```python
from build123d import *

# Parameters (mm, degrees)
SKETCH3_W           = 50
SKETCH3_H           = 100
BOSS_EXTRUDE1_DEPTH = 8
SKETCH3_3_R         = 8
SKETCH3_3_R_2       = 1.5
CUT_EXTRUDE2_DEPTH  = 10
SKETCH4_R           = 18.5
CUT_EXTRUDE3_DEPTH  = 4


with BuildPart() as part:
    # Sketch3 → Boss-Extrude1 (new body)
    with BuildSketch(Plane.XY):
        with Locations((0, 50)):
            Rectangle(SKETCH3_W, SKETCH3_H)
    extrude(amount=BOSS_EXTRUDE1_DEPTH)

    # Sketch3_3 → Cut-Extrude2 (cut)
    with BuildSketch(Plane.XY):
        with Locations(Location((0, 12.8, 0), (0, 0, 180))):
            Circle(SKETCH3_3_R)
        with Locations(Location((-7.75, 33.223393759, 0), (0, 0, 180))):
            Circle(SKETCH3_3_R_2)
        with Locations(Location((7.75, 33.223393759, 0), (0, 0, 180))):
            Circle(SKETCH3_3_R_2)
        with Locations(Location((-15.5, 19.8, 0), (0, 0, 180))):
            Circle(SKETCH3_3_R_2)
        with Locations(Location((-7.75, 6.376606241, 0), (0, 0, 180))):
            Circle(SKETCH3_3_R_2)
        with Locations(Location((7.75, 6.376606241, 0), (0, 0, 180))):
            Circle(SKETCH3_3_R_2)
        with Locations(Location((15.5, 19.8, 0), (0, 0, 180))):
            Circle(SKETCH3_3_R_2)
    extrude(amount=CUT_EXTRUDE2_DEPTH, mode=Mode.SUBTRACT)

    # Sketch4 → Cut-Extrude3 (cut)
    with BuildSketch(Plane.XY.offset(8)):
        with Locations((0, 19.8)):
            Circle(SKETCH4_R)
    extrude(amount=-CUT_EXTRUDE3_DEPTH, mode=Mode.SUBTRACT)


solid = part.part
```
CAD build for the part. Positions are in the model's coordinates, mm. A direction names the side the tool comes from. Round coordinates to 2 decimals unless told otherwise and drop trailing zeros. Loops run counter-clockwise (first coordinate to the right, second up) from the corner with the lowest first, then second, coordinate; pieces in that order, holes last. Notation, with made-up numbers: M -27,-33 L -11,-33 A12 cw -11,-29 Z; hole C -23,-10 d1. An arc over 180 degrees is marked long. Return JSON: item names as keys, results as strings. Group by question number.
(1) Saw through at A-A, the plane x = -15.5. List the corners of the cut face in (y, z), and give its area (3 significant figures).
(2) Saw through at C-C, the plane z = 6.25. List the corners of the cut face in (x, y), and give its area (3 significant figures).
(3) Mould opens along Y. For faces 3 (the flat face through (25, 49, 4)), 4 (the flat face through (0, 100, 4)), 5 (the cylindrical face through (8.856, 5.363, 1.972)), 6 (the cylindrical face through (-7.425, 34.688, 1.972)) say: +Y half, -Y half, draft (parallel to the pull), parting line (faces both ways), or undercut.
(4) Saw through at B-B, the plane y = 12.8. List the corners of the cut face in (x, z), and give its area (3 significant figures).
(5) Tool access for faces 1 (the cylindrical face through (-4.01, 1.74, 6.03)), 2 (the cylindrical face through (6.349, 17.668, 1.972)): list every direction of +Z, -Z, +X, -X, +Y, -Y with a clear straight run to the whole face (end or side of a thin tool).
(6) Wall check: probe 1 along Y at (x, z) = (0, 5.15); probe 2 along Y at (x, z) = (15.5, 1.55); probe 3 along X at (y, z) = (19.8, 2.2). Give the ranges that are in metal, low to high. Write a range as [from, to].
(7) Saw through at D-D, the plane z = 2. List the corners of the cut face in (x, y), and give its area (3 significant figures).
Answer list:
{
 "1": {"outline": "M 0,0 L 18.3,0 L 18.3,4 L 9.7,4 L 9.7,8 L 0,8 Z; M 21.3,0 L 100,0 L 100,8 L 29.9,8 L 29.9,4 L 21.3,4 Z", "area": "707 mm2"},
 "2": {"outline": "M -25,0 L 25,0 L 25,100 L -25,100 Z; hole C 0,19.8 d37", "area": "3,920 mm2"},
 "3": {"face 3": "draft", "face 4": "+Y half", "face 5": "undercut", "face 6": "undercut"},
 "4": {"outline": "M -25,0 L -8,0 L -8,4 L -17.12,4 L -17.12,8 L -25,8 Z; M 8,0 L 25,0 L 25,8 L 17.12,8 L 17.12,4 L 8,4 Z", "area": "199 mm2"},
 "5": {"face 1": "+Z", "face 2": "+Z, -Z"},
 "6": {"probe 1": "[0, 1.3], [38.3, 100]", "probe 2": "[0, 18.3], [21.3, 100]", "probe 3": "[-25, -17], [-14, -3.87], [3.87, 14], [17, 25]"},
 "7": {"outline": "M -25,0 L 25,0 L 25,100 L -25,100 Z; hole C -15.5,19.8 d3; hole C -7.75,6.38 d3; hole C -7.75,33.22 d3; hole C 0,12.8 d16; hole C 7.75,6.38 d3; hole C 7.75,33.22 d3; hole C 15.5,19.8 d3", "area": "4,760 mm2"}
}
